from build123d import *

# Parameters (mm, degrees)
CORTAR_EXTRUIR1_DEPTH      = 29.833660884
CORTAR_EXTRUIR1_DEPTH_BACK = 29.833660884
CROQUIS2_W                 = 3.8
CROQUIS2_H                 = 10.824175058
CROQUIS2_W_2               = 0.75
CROQUIS2_H_2               = 4
CORTAR_EXTRUIR2_DEPTH      = 29.580062981
CORTAR_EXTRUIR2_DEPTH_BACK = 29.580062981
CROQUIS4_W                 = 1.877516853
CROQUIS4_H                 = 6.743313928
CORTAR_EXTRUIR3_DEPTH      = 29.410077437
CORTAR_EXTRUIR3_DEPTH_BACK = 29.410077437
CROQUIS5_R                 = 1.5
TALADRO_ROSCADO_M31_D      = 2.5
TALADRO_ROSCADO_M31_DEPTH  = 14
TALADRO_ROSCADO_M31_TIP    = 0.751075774


with BuildPart() as part:
    # Croquis1 → Revolución1 (revolve)
    with BuildSketch(Plane.XY):
        with BuildLine():
            Line((0, 0), (0, 17.2))
            ThreePointArc((0, 17.2), (4.5, 21.7), (0, 26.2))
            Line((0, 26.2), (0, 27.6))
            ThreePointArc((0, 27.6), (5.65078016, 23.396668376), (3.25, 16.775824942))
            Line((3.25, 16.775824942), (3.25, 4))
            Line((3.25, 4), (4, 4))
            Line((4, 4), (4, 0))
            Line((4, 0), (0, 0))
        make_face()
    revolve(axis=Axis((0, 0, 0), (0, 1, 0)))

    # Croquis2 → Cortar-Extruir1 (cut, two sides: drawn at the far end of the back side and taken through both)
    with BuildSketch(Plane(origin=(0, 0, 0), x_dir=(0, 0, -1), z_dir=(1, 0, 0)).offset(-CORTAR_EXTRUIR1_DEPTH_BACK)):
        with Locations((-4, 22.187912471)):
            Rectangle(CROQUIS2_W, CROQUIS2_H)
        with Locations((4, 22.187912471)):
            Rectangle(CROQUIS2_W, CROQUIS2_H)
        Polygon((-3.25, 15.625824942), (-2.1, 16.775824942), (-3.25, 16.775824942), align=None)
        Polygon((3.25, 16.775824942), (2.1, 16.775824942), (3.25, 15.625824942), align=None)
        with Locations((3.625, 2)):
            Rectangle(CROQUIS2_W_2, CROQUIS2_H_2)
        with Locations((-3.625, 2)):
            Rectangle(CROQUIS2_W_2, CROQUIS2_H_2)
    extrude(amount=CORTAR_EXTRUIR1_DEPTH + CORTAR_EXTRUIR1_DEPTH_BACK, mode=Mode.SUBTRACT)

    # Croquis3 → Revolución2 (revolve)
    with BuildSketch(Plane.XY):
        with BuildLine():
            Line((0, 26.2), (0, 17.2))
            ThreePointArc((0, 17.2), (-4.5, 21.7), (0, 26.2))
        make_face()
    revolve(axis=Axis((0, 26.2, 0), (0, -1, 0)))

    # Croquis4 → Cortar-Extruir2 (cut, two sides: drawn at the far end of the back side and taken through both)
    with BuildSketch(Plane(origin=(0, 0, 0), x_dir=(0, 0, -1), z_dir=(1, 0, 0)).offset(-CORTAR_EXTRUIR2_DEPTH_BACK)):
        with Locations((-3.938758427, 21.717554998)):
            Rectangle(CROQUIS4_W, CROQUIS4_H)
        with Locations((3.938758427, 21.717554998)):
            Rectangle(CROQUIS4_W, CROQUIS4_H)
    extrude(amount=CORTAR_EXTRUIR2_DEPTH + CORTAR_EXTRUIR2_DEPTH_BACK, mode=Mode.SUBTRACT)

    # Croquis5 → Cortar-Extruir3 (cut, two sides: drawn at the far end of the back side and taken through both)
    with BuildSketch(Plane.XY.offset(-CORTAR_EXTRUIR3_DEPTH_BACK)):
        with Locations((0, 21.7)):
            Circle(CROQUIS5_R)
    extrude(amount=CORTAR_EXTRUIR3_DEPTH + CORTAR_EXTRUIR3_DEPTH_BACK, mode=Mode.SUBTRACT)

    # Taladro roscado M31
    with Locations(Plane(origin=(0, 0, 0), x_dir=(-1, 0, 0), z_dir=(0, -1, 0))):
        with Locations((0, 0)):
            Hole(TALADRO_ROSCADO_M31_D / 2, depth=TALADRO_ROSCADO_M31_DEPTH)
            with Locations((0, 0, -(TALADRO_ROSCADO_M31_DEPTH + TALADRO_ROSCADO_M31_TIP / 2))):  # 118° drill point
                Cone(0, TALADRO_ROSCADO_M31_D / 2, TALADRO_ROSCADO_M31_TIP, mode=Mode.SUBTRACT)


solid = part.part
Can you work these out from the model? Positions are in its coordinate system, mm. A direction names the side the tool comes from. Coordinates: 2 decimals unless noted, no trailing zeros. Loops run counter-clockwise (first coordinate to the right, second up) from the corner with the lowest first, then second, coordinate; pieces in that order, holes last. Notation, with made-up numbers: M -1,66 L 58,66 A32 cw 58,96 Z; hole C 58,-10 d7. An arc over 180 degrees is marked long. Return JSON: item names as keys, results as strings. Group by question number.
Item 1: On a 3-axis mill with a long thin cutter (end or side, diameter ignored), from which of +Z, -Z, +X, -X, +Y, -Y can I reach the whole of each face in a straight line? I mean faces 4 (the flat face through (3.5, 4, 0)), 5 (the flat face through (-0.035, 16.321, 2.555)), 6 (the flat face through (-4, 23, -2.1)), 7 (the cylindrical face through (4, 2, 0)). Say none if no direction works.
Item 2: Imagine slicing it at D-D (x = -3). Please give me the cut outline in (y, z).
Item 3: Imagine slicing it at A-A (z = 2.75). Please give me the cut outline in (x, y).
Item 4: I'm going to push flat-ended pins straight in: pin 1 Ø5 at (x, y) = (-2, 20.5) entering from -Z; pin 2 Ø2.5 at (x, y) = (0, 21.7) entering from -Z; pin 3 Ø1 at (x, y) = (-3.5, 23.5) entering from -Z; pin 4 Ø2 at (x, y) = (-1, 23) entering from +Z. Where does each tip first touch, or does it pass through?
Item 5: Imagine slicing it at B-B (y = 21.7). Please give me the cut outline in (x, z), and give its area (3 significant figures).
Item 6: Imagine slicing it at C-C (y = 5). Please give me the cut outline in (x, z), and give its area (3 significant figures).
Item 7: If I drill on L1, parallel to Z at x = 0, y = 10.75; L2, parallel to Z at x = -3, y = 5; L3, parallel to Y at x = 1, z = -2.25, over which ranges is the centre line in solid material (lowest first)? Write a range as from..to.
Item 8: Thinking about a two-plate mould opening in Z: for faces 1 (the flat face through (-3.5, 4, 0)), 2 (the flat face through (0, 2, -3.25)), 3 (the conical face through (0.05, 14.62, 0.21)), which applies, released by +Z, released by -Z, zero draft, split by the parting line, or undercut?
Verdict:
{
 "1": {"face 4": "+X", "face 5": "+Z, +X, -X", "face 6": "-Z", "face 7": "+X, -Y"},
 "2": {"outline": "M 0,-2.65 L 4,-2.65 L 4,-1.25 L 16.78,-1.25 A5.08 ccw 17.07,-2.1 L 19.08,-2.1 A3.35 ccw 20.2,-3 L 23.2,-3 A3.35 ccw 24.32,-2.1 L 26.33,-2.1 A5.08 ccw 26.33,2.1 L 24.32,2.1 A3.35 ccw 23.2,3 L 20.2,3 A3.35 ccw 19.08,2.1 L 17.07,2.1 A5.08 ccw 16.78,1.25 L 4,1.25 L 4,2.65 L 0,2.65 Z"},
 "3": {"outline": "C 0,21.7 d7.12; M -2.9,0 L 2.9,0 L 2.9,4 L 1.73,4 L 1.73,16.13 L -1.73,16.13 L -1.73,4 L -2.9,4 Z; hole C 0,21.7 d3"},
 "4": {"pin 1": "stops at z = -3", "pin 2": "passes through", "pin 3": "stops at z = -2.91", "pin 4": "stops at z = 3"},
 "5": {"outline": "M -5.51,-2.1 L -3.98,-2.1 A4.5 ccw -3.35,-3 L -1.5,-3 L -1.5,3 L -3.35,3 A4.5 ccw -3.98,2.1 L -5.51,2.1 A5.9 ccw Z; M 1.5,-3 L 3.35,-3 A4.5 ccw 3.98,-2.1 L 5.51,-2.1 A5.9 ccw 5.51,2.1 L 3.98,2.1 A4.5 ccw 3.35,3 L 1.5,3 Z", "area": "43.8 mm^2"},
 "6": {"outline": "C 0,0 d6.5; hole C 0,0 d2.5", "area": "28.3 mm^2"},
 "7": {"L1": "z = -3.25..-1.25, 1.25..3.25", "L2": "z = -1.25..1.25", "L3": "y = 0..16.63, 17.93..20.58, 22.82..25.47"},
 "8": {"face 1": "zero draft", "face 2": "released by -Z", "face 3": "undercut"}
}
